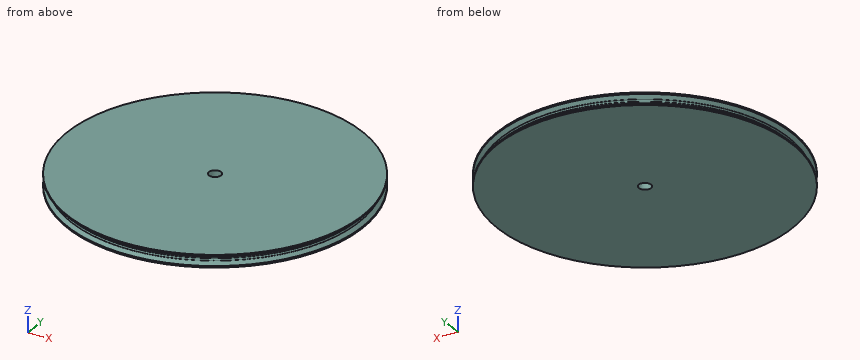
```python
from build123d import *


with BuildPart() as part:
    # Sketch1 → Revolve1 (revolve)
    with BuildSketch(Plane(origin=(0, 0, 0), x_dir=(1, 0, 0), z_dir=(0, 1, 0))):
        with BuildLine():
            Line((6.35, 6.35), (152.4, 6.35))
            Line((152.4, 6.35), (152.4, 4.85))
            Line((152.4, 4.85), (148.8, 1.25))
            ThreePointArc((148.8, 1.25), (147.55, 0), (148.8, -1.25))
            Line((148.8, -1.25), (152.4, -4.85))
            Line((152.4, -4.85), (152.4, -6.35))
            Line((152.4, -6.35), (6.35, -6.35))
            Line((6.35, -6.35), (6.35, 6.35))
        make_face()
    revolve(axis=Axis((0, 0, 6.35), (0, 0, -1)))


solid = part.part
```
Verification items for the finished model (mm, model axes). Round coordinates to 2 decimals unless told otherwise and drop trailing zeros. Order: outer loops, then holes, each group sorted by start corner. A loop starts at its lowest first (then second) coordinate and runs counter-clockwise, first axis right, second up. Notation, with made-up numbers: (29, 71.5) -> (56, 71.5) arc R15 ccw to (56, 75.5) -> close; hole circle Ø7 at (78, 4). An arc over 180 degrees is marked (long way). Put each result on its own line as item: value. Start each with the question number.
(1) Depth check by flat-ended pin: pin 1 Ø6 at (y, z) = (90, -4.5) entering from +X; pin 2 Ø10 at (x, y) = (0, 0) entering from +Z; pin 3 Ø2 at (x, z) = (16, -4) entering from -Y; pin 4 Ø5 at (y, z) = (-115.5, 3.5) entering from -X. Enter the tip coordinate at first touch or a pass-through.
(2) Section check A-A (y = 0). Enter the section's corners in (x, z), then the cut area to 3 significant figures.
(3) Material ranges on line 1 along Y through (x, z) = (0, -1.75); line 2 along Y through (x, z) = (0, -0.25), recorded low to high.
Completed:
1. pin 1: stops at x = 125.11
1. pin 2: passes through
1. pin 3: stops at y = -151.61
1. pin 4: stops at x = -101.82
2. outline: (-152.4, -6.35) -> (-6.35, -6.35) -> (-6.35, 6.35) -> (-152.4, 6.35) -> (-152.4, 4.85) -> (-148.8, 1.25) arc R1.25 cw to (-148.8, -1.25) -> (-152.4, -4.85) -> close; (6.35, -6.35) -> (152.4, -6.35) -> (152.4, -4.85) -> (148.8, -1.25) arc R1.25 cw to (148.8, 1.25) -> (152.4, 4.85) -> (152.4, 6.35) -> (6.35, 6.35) -> close
2. area: 3,660 mm2
3. line 1: y = -149.3 to -6.35, 6.35 to 149.3
3. line 2: y = -147.58 to -6.35, 6.35 to 147.58
